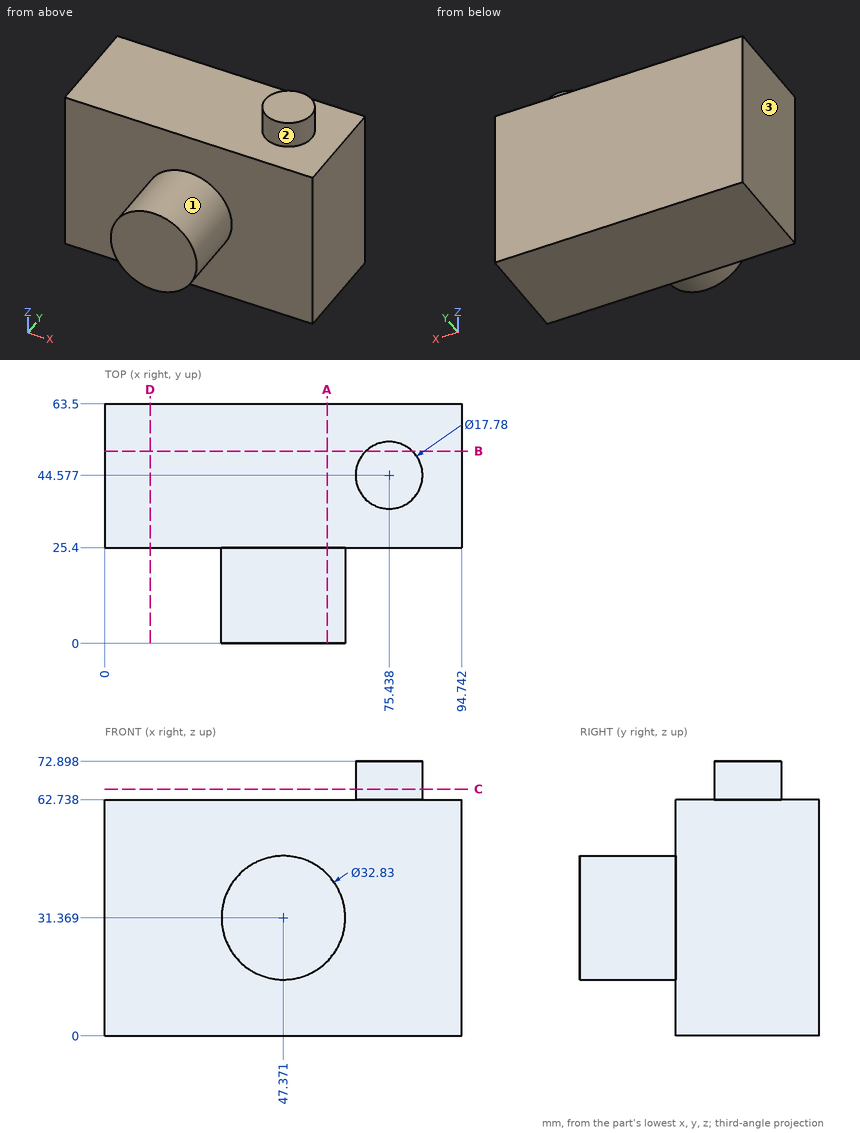
Answer from the drawing. Dimensions are ordinates in mm from the lowest x, y and z of the part. A direction names the side the tool comes from. Round coordinates to 2 decimals unless told otherwise and drop trailing zeros. Write each loop counter-clockwise with the first axis right and the second up, starting at its lowest first coordinate (ties: lowest second). Pieces come first, ordered by that corner, then holes. Notation, with made-up numbers: M 72,31 L 126,31 A14 ccw 126,54 Z; hole C 59,-11 d11. An arc over 180 degrees is marked long. Write each question's results on one line, items separated by ' | '. Start each with the question number.
Item 1: Find section B-B on y = 51. Write down the section's boundary in (x, z), and give its area (3 significant figures).
Item 2: Given pin 1 Ø4 at (x, y) = (32, 19.5) entering from +Z; pin 2 Ø2 at (x, z) = (29, 29.5) entering from -Y; pin 3 Ø10 at (x, y) = (44, 17.5) entering from +Z, each flat-ended and moving along its own axis, determine where each tip first touches the part or whether it passes through.
Item 3: Which of the six approach directions +Z, -Z, +X, -X, +Y, -Y give full straight-line access (tool end or side, diameter ignored) to the marked faces 1, 2 and 3?
Item 4: Find section A-A on x = 59. Write down the section's boundary in (y, z).
Item 5: Straight lines are drawn through the part: probe 1 along Y at (x, z) = (29, 6); probe 2 along Z at (x, y) = (22, 27.5); probe 3 along X at (y, z) = (17, 33.5) (3 decimals). For each, find the intervals that lie inside material, in ascending order.
Item 6: Find section D-D on x = 12. Write down the section's boundary in (y, z).
Item 7: Find section C-C on z = 65.5. Write down the section's boundary in (x, y).
Answer block:
1) outline: M 0,0 L 94.74,0 L 94.74,62.74 L 81.58,62.74 L 81.58,72.9 L 69.29,72.9 L 69.29,62.74 L 0,62.74 Z | area: 6,070 mm²
2) pin 1: stops at z = 40.89 | pin 2: stops at y = 25.4 | pin 3: stops at z = 47.78
3) face 1: -Y | face 2: +Z | face 3: +Z, -Z, -X, +Y, -Y
4) outline: M 0,19.78 L 25.4,19.78 L 25.4,0 L 63.5,0 L 63.5,62.74 L 25.4,62.74 L 25.4,42.95 L 0,42.95 Z
5) probe 1: y = 25.4 to 63.5 | probe 2: z = 0 to 62.74 | probe 3: x = 31.095 to 63.647
6) outline: M 25.4,0 L 63.5,0 L 63.5,62.74 L 25.4,62.74 Z
7) outline: C 75.44,44.58 d17.78
